Check sheet for the modelled part. Datum: model origin and axes. Units: mm. A direction names the side the tool comes from. Round coordinates to 2 decimals unless told otherwise and drop trailing zeros. Loops run counter-clockwise (first coordinate to the right, second up) from the corner with the lowest first, then second, coordinate; pieces in that order, holes last. Notation, with made-up numbers: (42.5, -2) - (80.5, -2) arc R6 ccw to (80.5, 4) - close; hole circle Ø10 at (60, 40.25). An arc over 180 degrees is marked (long way). Return JSON: item names as keys, results as strings.
from build123d import *

# Parameters (mm, degrees)
BASE_EXTRUDE_DEPTH   = 2
HOLES_R              = 1.15
HOLES_CUT_DEPTH      = 3
INSIDE_W             = 85.5
INSIDE_H             = 58
INSIDE_EXTRUDE_DEPTH = 2


with BuildPart() as part:
    # Base → Base Extrude (new body)
    with BuildSketch(Plane(origin=(0, 0, 0), x_dir=(1, 0, 0), z_dir=(0, 1, 0))):
        with BuildLine():
            Line((6, 0), (84, 0))
            ThreePointArc((84, 0), (87, -3), (90, 0))
            Line((90, 0), (90, 62.5))
            ThreePointArc((90, 62.5), (87, 65.5), (84, 62.5))
            Line((84, 62.5), (6, 62.5))
            ThreePointArc((6, 62.5), (3, 65.5), (0, 62.5))
            Line((0, 62.5), (0, 0))
            ThreePointArc((0, 0), (3, -3), (6, 0))
        make_face()
    extrude(amount=BASE_EXTRUDE_DEPTH)

    # Holes → Holes Cut (cut, through all)
    with BuildSketch(Plane(origin=(0, 2, 0), x_dir=(1, 0, 0), z_dir=(0, 1, 0))):
        with Locations((3, 62.5)):
            Circle(HOLES_R)
        with Locations((87, 62.5)):
            Circle(HOLES_R)
        with Locations((87, 0)):
            Circle(HOLES_R)
        with Locations((3, 0)):
            Circle(HOLES_R)
    extrude(amount=-HOLES_CUT_DEPTH, mode=Mode.SUBTRACT)

    # Inside → Inside Extrude (add)
    with BuildSketch(Plane.XZ):
        with Locations((45, -31.25)):
            Rectangle(INSIDE_W, INSIDE_H)
    extrude(amount=INSIDE_EXTRUDE_DEPTH)


solid = part.part
Q1. Depth check by flat-ended pin: P1, Ø2, axis at x = 87, z = -62.5, coming from the -Y side; P2, Ø1.6, axis at x = 43.5, y = 1.5, coming from the -Z side; P3, Ø2, axis at y = -0.5, z = -27, coming from the -X side; P4, Ø0.6, axis at x = 37, y = 1, coming from the +Z side. Enter the tip coordinate at first touch or a pass-through.
Answer key:
{"P1": "passes through", "P2": "stops at z = -62.5", "P3": "stops at x = 0", "P4": "stops at z = 0"}
Q2. Draft check along Z on faces 6 (the face through (44, -2, -31)), 7 (the face through (3.1, 1, -65.5)), 8 (the face through (86.85, 1.01, -63.64)). Enter one of: released by +Z, released by -Z, zero draft, split by the parting line, or undercut.
Answer key:
{"face 6": "zero draft", "face 7": "released by -Z", "face 8": "undercut"}
Q3. Sectioned sample at B-B (x = 45.5). Enter the section's corners in (y, z).
Answer key:
{"outline": "(-2, -60.25) - (0, -60.25) - (0, -62.5) - (2, -62.5) - (2, 0) - (0, 0) - (0, -2.25) - (-2, -2.25) - close"}
Q4. Sectioned sample at A-A (z = -5.5). Enter the section's corners in (x, y).
Answer key:
{"outline": "(0, 0) - (2.25, 0) - (2.25, -2) - (87.75, -2) - (87.75, 0) - (90, 0) - (90, 2) - (0, 2) - close"}
Q5. Tool access check on faces 1 (the face through (44, -1, -60.25)), 2 (the face through (44, 1, 0)), 3 (the face through (2.25, -1, -32)), 4 (the face through (46, 1, -62.5)), 5 (the face through (87.75, -1, -32)). Record the directions out of +Z, -Z, +X, -X, +Y, -Y that give a thin tool (end or side, any length) a straight path to the whole face; none if there is none.
Answer key:
{"face 1": "-Z, +X, -X, -Y", "face 2": "+Z, +Y, -Y", "face 3": "+Z, -Z, -X, -Y", "face 4": "-Z, +Y, -Y", "face 5": "+Z, -Z, +X, -Y"}
Q6. Scan lines: probe 1 along Z at (x, y) = (87, 1); probe 2 along X at (y, z) = (0.5, 0.5); probe 3 along Z at (x, y) = (5, -1.25). Record each from-to range of solid material in increasing order. Write a range as [from, to].
Answer key:
{"probe 1": "z = [-65.5, -63.65], [-61.35, -1.15], [1.15, 3]", "probe 2": "x = [0.04, 1.96], [4.04, 5.96], [84.04, 85.96], [88.04, 89.96]", "probe 3": "z = [-60.25, -2.25]"}
